```python
from build123d import *

# Parameters (mm, degrees)
BOSS_EXTRUDE1_DEPTH = 4
CUT_EXTRUDE1_DEPTH  = 2
CUT_EXTRUDE2_DEPTH  = 2


with BuildPart() as part:
    # Sketch1 → Boss-Extrude1 (new body)
    with BuildSketch(Plane(origin=(0, 0, 0), x_dir=(1, 0, 0), z_dir=(0, 1, 0))):
        Polygon((-25, 50.39), (33.74, -25), (33.74, -45), (-25, -45), align=None)
    extrude(amount=BOSS_EXTRUDE1_DEPTH)

    # Sketch2 → Cut-Extrude1 (cut)
    with BuildSketch(Plane(origin=(0, 4, 0), x_dir=(1, 0, 0), z_dir=(0, 1, 0))):
        Polygon((-23, -2.0971477), (7.121683168, -7.35422298), (9.012903271, 3.481979608), (-21.498978305, 8.961494434), align=None)
    extrude(amount=-CUT_EXTRUDE1_DEPTH, mode=Mode.SUBTRACT)

    # Sketch4 → Cut-Extrude2 (cut)
    with BuildSketch(Plane(origin=(0, 4, 0), x_dir=(1, 0, 0), z_dir=(0, 1, 0))):
        Polygon((-4.867869217, -9.85422298), (25.219953937, -17.319000128), (22.558813085, -27.992253117), (-7.520354429, -20.492674354), align=None)
    extrude(amount=-CUT_EXTRUDE2_DEPTH, mode=Mode.SUBTRACT)


solid = part.part
```
Check sheet for the modelled part. Datum: model origin and axes. Units: mm. A direction names the side the tool comes from. Give positions to 0.01 mm unless a question says otherwise; leave off trailing zeros. Order: outer loops, then holes, each group sorted by start corner. A loop starts at its lowest first (then second) coordinate and runs counter-clockwise, first axis right, second up. Notation, with made-up numbers: (4, 78.5) -> (53, 78.5) arc R18 ccw to (53, 90.5) -> close; hole circle Ø3 at (21, 17.25). An arc over 180 degrees is marked (long way). Use CSV: the item, a comma, the result in double quotes. Start each with the question number.
1) Sectioned sample at A-A, the plane y = 3.15. Record the boundary of the cut face in (x, z).
2) Sectioned sample at B-B, the plane z = 13. Record the boundary of the cut face in (x, y).
3) Set-up check for faces 1 (the face through (3.96, 1.97, -13.22)), 2 (the face through (-7, 2, -1)): record each of +Z, -Z, +X, -X, +Y, -Y from which the full face is reachable in a straight line by a thin tool's end or side.
4) Sectioned sample at D-D, the plane z = -6. Record the boundary of the cut face in (x, y), plus the area to 3 significant figures.
5) Mould release check, pull along X, two halves, no side actions. Record for faces 3 (the face through (8.054, 3.014, 2.012)), 4 (the face through (5, 2, 45)), 5 (the face through (-25, 2, -2)): released by +X, released by -X, zero draft, split by the parting line, or undercut.
6) Sectioned sample at C-C, the plane x = -2.5. Record the boundary of the cut face in (y, z).
7) Go/stop test with flat-tipped pins: P1, Ø18, axis at x = -4, z = -4, coming from the +Y side; P2, Ø1.5, axis at y = 3, z = -21.5, coming from the +X side; P3, Ø1.5, axis at x = 14.5, z = 17, coming from the +Y side. Record where each tip stops, or that it passes through.
8) Material ranges on line 1 (Z direction, x = 2.5, y = 3.65); line 2 (Y direction, x = -11.5, z = 3); line 3 (Z direction, x = 17.5, y = 2.4), recorded low to high. Write a range as from..to.
Recorded:
1,outline,"(-25, -50.39) -> (33.74, 25) -> (33.74, 45) -> (-25, 45) -> close; hole (-23, 2.1) -> (-21.5, -8.96) -> (9.01, -3.48) -> (7.12, 7.35) -> close; hole (-7.52, 20.49) -> (-4.87, 9.85) -> (25.22, 17.32) -> (22.56, 27.99) -> close"
2,outline,"(-25, 0) -> (24.39, 0) -> (24.39, 4) -> (7.81, 4) -> (7.81, 2) -> (-5.65, 2) -> (-5.65, 4) -> (-25, 4) -> close"
3,face 1,"-Z, +X, +Y, -Y"
3,face 2,"+Y"
4,outline,"(-25, 0) -> (9.59, 0) -> (9.59, 4) -> (-5.01, 4) -> (-5.01, 2) -> (-21.9, 2) -> (-21.9, 4) -> (-25, 4) -> close"
4,area,"105 mm2"
5,face 3,"undercut"
5,face 4,"zero draft"
5,face 5,"released by -X"
6,outline,"(0, -21.51) -> (4, -21.51) -> (4, -5.55) -> (2, -5.55) -> (2, 5.67) -> (4, 5.67) -> (4, 10.44) -> (2, 10.44) -> (2, 21.74) -> (4, 21.74) -> (4, 45) -> (0, 45) -> close"
7,P1,"y = 4"
7,P2,"x = -1.91"
7,P3,"y = 2"
8,line 1,"-15.1..-4.65, 6.55..11.68, 22.99..45"
8,line 2,"0..2"
8,line 3,"4.16..15.4, 26.73..45"
